For this review, take the finished solid that the model builds, in its own axes (mm). A direction names the side the tool comes from. Round coordinates to 2 decimals unless told otherwise and drop trailing zeros. Write each loop counter-clockwise with the first axis right and the second up, starting at its lowest first coordinate (ties: lowest second). Pieces come first, ordered by that corner, then holes.
from build123d import *

# Parameters (mm, degrees)
BOSS_EXTRUDE1_DEPTH = 60
BOSS_EXTRUDE2_DEPTH = 42
CUT_EXTRUDE1_DEPTH  = 42
SKETCH4_R           = 15
SKETCH4_R_2         = 10
BOSS_EXTRUDE4_DEPTH = 18
CUT_EXTRUDE2_START  = -10
SKETCH4_2_R         = 10
CUT_EXTRUDE2_DEPTH  = 10
CUT_EXTRUDE3_START  = -127
SKETCH5_W           = 40
SKETCH5_H           = 20
CUT_EXTRUDE3_DEPTH  = 127
SKETCH6_R           = 6.5
CUT_EXTRUDE4_DEPTH  = 183
SKETCH7_R           = 4
CUT_EXTRUDE5_DEPTH  = 245
FILLET1_R           = 3
FILLET2_R           = 5
BOSS_EXTRUDE6_DEPTH = 22


with BuildPart() as part:
    # Sketch1 → Boss-Extrude1 (new body)
    with BuildSketch(Plane.XY):
        Polygon((170, 20), (130, 20), (0, 20), (0, 0), (170, 0), align=None)
    extrude(amount=BOSS_EXTRUDE1_DEPTH)

    # Sketch1<3> → Boss-Extrude2 (add)
    with BuildSketch(Plane.XY):
        with BuildLine():
            Line((35, 60), (35, 20))
            Line((35, 20), (45, 20))
            Line((45, 20), (45, 60))
            ThreePointArc((45, 60), (49.292505485, 81.301408404), (61.5, 99.277856357))
            ThreePointArc((61.5, 99.277856357), (66.936491673, 100.316914371), (70, 95.707142143))
            Line((70, 95.707142143), (70, 20))
            Line((70, 20), (100, 20))
            Line((100, 20), (78, 45))
            Line((78, 45), (78, 85))
            Line((78, 85), (130, 85))
            Line((130, 85), (130, 157))
            Line((130, 157), (115, 157))
            Line((115, 157), (115, 175))
            Line((115, 175), (85, 175))
            Line((85, 175), (85, 157))
            Line((85, 157), (70, 157))
            Line((70, 157), (70, 117.662812973))
            ThreePointArc((70, 117.662812973), (44.434723073, 93.726843908), (35, 60))
        make_face()
        Polygon((100, 20), (130, 20), (130, 45), (122, 45), align=None)
    extrude(amount=BOSS_EXTRUDE2_DEPTH)

    # Sketch3 → Cut-Extrude1 (cut)
    with BuildSketch(Plane(origin=(115, 0, 0), x_dir=(0, 0, -1), z_dir=(1, 0, 0))):
        Polygon((-42, 157), (7.234036257, 157), (7.234036257, 179.627454065), (-54.634398112, 179.627454065), (-54.634398112, 157), align=None)
    extrude(amount=-CUT_EXTRUDE1_DEPTH, mode=Mode.SUBTRACT)

    # Sketch4 → Boss-Extrude4 (add)
    with BuildSketch(Plane(origin=(0, 157, 0), x_dir=(1, 0, 0), z_dir=(0, 1, 0))):
        with Locations((100, -21)):
            Circle(SKETCH4_R)
        with Locations(Location((100, -21, 0), (0, 0, 180))):
            Circle(SKETCH4_R_2, mode=Mode.SUBTRACT)
    extrude(amount=BOSS_EXTRUDE4_DEPTH)

    # Sketch4<2> → Cut-Extrude2 (cut)
    with BuildSketch(Plane(origin=(0, 157, 0), x_dir=(1, 0, 0), z_dir=(0, 1, 0)).offset(CUT_EXTRUDE2_START)):
        with Locations(Location((100, -21, 0), (0, 0, 180))):
            Circle(SKETCH4_2_R)
    extrude(amount=CUT_EXTRUDE2_DEPTH, mode=Mode.SUBTRACT)

    # Sketch5 → Cut-Extrude3 (cut)
    with BuildSketch(Plane(origin=(0, 147, 0), x_dir=(1, 0, 0), z_dir=(0, 1, 0)).offset(CUT_EXTRUDE3_START)):
        with Locations((100, -21)):
            Rectangle(SKETCH5_W, SKETCH5_H)
    extrude(amount=CUT_EXTRUDE3_DEPTH, mode=Mode.SUBTRACT)

    # Sketch6 → Cut-Extrude4 (cut)
    with BuildSketch(Plane(origin=(0, 20, 0), x_dir=(1, 0, 0), z_dir=(0, 1, 0))):
        with Locations(Location((15, -30, 0), (0, 0, 180))):
            Circle(SKETCH6_R)
        with Locations(Location((155, -30, 0), (0, 0, 180))):
            Circle(SKETCH6_R)
    extrude(amount=-CUT_EXTRUDE4_DEPTH, mode=Mode.SUBTRACT)

    # Sketch7 → Cut-Extrude5 (cut)
    with BuildSketch(Plane(origin=(130, 0, 0), x_dir=(0, 0, -1), z_dir=(1, 0, 0))):
        with Locations((-20, 140)):
            Circle(SKETCH7_R)
    extrude(amount=-CUT_EXTRUDE5_DEPTH, mode=Mode.SUBTRACT)

    # Fillet1
    # the kernel refuses this fillet: 3 mm, written as the material it adds along each edge
    with BuildSketch(Plane(origin=(100, 20, 42), x_dir=(0, 0, 1), z_dir=(1, 0, 0))) as fillet1_piece_1_section:
        with BuildLine():
            CenterArc((FILLET1_R, -FILLET1_R), FILLET1_R, 90, 90)
            Line((0, -FILLET1_R), (0, 0))
            Line((0, 0), (FILLET1_R, 0))
        make_face()
    fillet1_piece_1 = extrude(amount=30, mode=Mode.PRIVATE)
    fillet1_piece_1 = split(fillet1_piece_1, bisect_by=Plane(origin=(107.006094621, 27.96147116, 42.686468699), z_dir=(0.7507135169227557, -0.6606278948920244, 0)), keep=Keep.TOP, mode=Mode.PRIVATE)
    add(fillet1_piece_1)
    with BuildSketch(Plane(origin=(78, 85, 0), x_dir=(0, -1, 0), z_dir=(0, 0, 1))) as fillet1_piece_2_section:
        with BuildLine():
            CenterArc((FILLET1_R, FILLET1_R), FILLET1_R, 180, 90)
            Line((0, FILLET1_R), (0, 0))
            Line((0, 0), (FILLET1_R, 0))
        make_face()
    fillet1_piece_2 = extrude(amount=42, mode=Mode.PRIVATE)
    fillet1_piece_2 = split(fillet1_piece_2, bisect_by=Plane(origin=(78.588320005, 84.284989696, 11), z_dir=(0, 0, -1)), keep=Keep.TOP, mode=Mode.PRIVATE)
    fillet1_piece_2 = split(fillet1_piece_2, bisect_by=Plane(origin=(80, 84.284989696, 5.5), z_dir=(-1, 0, 0)), keep=Keep.TOP, mode=Mode.PRIVATE)
    add(fillet1_piece_2)
    with BuildSketch(Plane(origin=(78, 85, 0), x_dir=(0, -1, 0), z_dir=(0, 0, 1))) as fillet1_piece_3_section:
        with BuildLine():
            CenterArc((FILLET1_R, FILLET1_R), FILLET1_R, 180, 90)
            Line((0, FILLET1_R), (0, 0))
            Line((0, 0), (FILLET1_R, 0))
        make_face()
    fillet1_piece_3 = extrude(amount=42, mode=Mode.PRIVATE)
    fillet1_piece_3 = split(fillet1_piece_3, bisect_by=Plane(origin=(80.37802851, 84.990607918, 11), z_dir=(0, 0, -1)), keep=Keep.TOP, mode=Mode.PRIVATE)
    fillet1_piece_3 = split(fillet1_piece_3, bisect_by=Plane(origin=(80, 84.990607918, 5.5), z_dir=(1, 0, 0)), keep=Keep.TOP, mode=Mode.PRIVATE)
    add(fillet1_piece_3)
    with BuildSketch(Plane(origin=(78, 85, 0), x_dir=(0, -1, 0), z_dir=(0, 0, 1))) as fillet1_piece_4_section:
        with BuildLine():
            CenterArc((FILLET1_R, FILLET1_R), FILLET1_R, 180, 90)
            Line((0, FILLET1_R), (0, 0))
            Line((0, 0), (FILLET1_R, 0))
        make_face()
    fillet1_piece_4 = extrude(amount=42, mode=Mode.PRIVATE)
    fillet1_piece_4 = split(fillet1_piece_4, bisect_by=Plane(origin=(78.588320005, 84.284989696, 11), z_dir=(0, 0, 1)), keep=Keep.TOP, mode=Mode.PRIVATE)
    fillet1_piece_4 = split(fillet1_piece_4, bisect_by=Plane(origin=(80, 84.284989696, 21), z_dir=(-1, 0, 0)), keep=Keep.TOP, mode=Mode.PRIVATE)
    fillet1_piece_4 = split(fillet1_piece_4, bisect_by=Plane(origin=(78.588320005, 84.284989696, 31), z_dir=(0, 0, -1)), keep=Keep.TOP, mode=Mode.PRIVATE)
    add(fillet1_piece_4)
    with BuildSketch(Plane(origin=(78, 85, 0), x_dir=(0, -1, 0), z_dir=(0, 0, 1))) as fillet1_piece_5_section:
        with BuildLine():
            CenterArc((FILLET1_R, FILLET1_R), FILLET1_R, 180, 90)
            Line((0, FILLET1_R), (0, 0))
            Line((0, 0), (FILLET1_R, 0))
        make_face()
    fillet1_piece_5 = extrude(amount=42, mode=Mode.PRIVATE)
    fillet1_piece_5 = split(fillet1_piece_5, bisect_by=Plane(origin=(80, 84.284989696, 36.5), z_dir=(-1, 0, 0)), keep=Keep.TOP, mode=Mode.PRIVATE)
    fillet1_piece_5 = split(fillet1_piece_5, bisect_by=Plane(origin=(78.588320005, 84.284989696, 31), z_dir=(0, 0, 1)), keep=Keep.TOP, mode=Mode.PRIVATE)
    add(fillet1_piece_5)
    with BuildSketch(Plane(origin=(78, 85, 0), x_dir=(0, -1, 0), z_dir=(0, 0, 1))) as fillet1_piece_6_section:
        with BuildLine():
            CenterArc((FILLET1_R, FILLET1_R), FILLET1_R, 180, 90)
            Line((0, FILLET1_R), (0, 0))
            Line((0, 0), (FILLET1_R, 0))
        make_face()
    fillet1_piece_6 = extrude(amount=42, mode=Mode.PRIVATE)
    fillet1_piece_6 = split(fillet1_piece_6, bisect_by=Plane(origin=(80, 84.990607918, 36.5), z_dir=(1, 0, 0)), keep=Keep.TOP, mode=Mode.PRIVATE)
    fillet1_piece_6 = split(fillet1_piece_6, bisect_by=Plane(origin=(80.37802851, 84.990607918, 31), z_dir=(0, 0, 1)), keep=Keep.TOP, mode=Mode.PRIVATE)
    add(fillet1_piece_6)
    with BuildSketch(Plane(origin=(130, 20, 0), x_dir=(1, 0, 0), z_dir=(0, 0, 1))) as fillet1_piece_7:
        with BuildLine():
            CenterArc((FILLET1_R, FILLET1_R), FILLET1_R, 180, 90)
            Line((0, FILLET1_R), (0, 0))
            Line((0, 0), (FILLET1_R, 0))
        make_face()
    extrude(amount=42)
    with BuildSketch(Plane(origin=(70, 20, 42), x_dir=(0, 0, 1), z_dir=(1, 0, 0))) as fillet1_piece_8_section:
        with BuildLine():
            CenterArc((FILLET1_R, -FILLET1_R), FILLET1_R, 90, 90)
            Line((0, -FILLET1_R), (0, 0))
            Line((0, 0), (FILLET1_R, 0))
        make_face()
    fillet1_piece_8 = extrude(amount=30, mode=Mode.PRIVATE)
    fillet1_piece_8 = split(fillet1_piece_8, bisect_by=Plane(origin=(92.993905379, 27.96147116, 42.686468699), z_dir=(-0.7507135169227557, -0.6606278948920244, 0)), keep=Keep.TOP, mode=Mode.PRIVATE)
    add(fillet1_piece_8)
    with BuildSketch(Plane(origin=(35, 20, 0), x_dir=(-1, 0, 0), z_dir=(0, 0, 1))) as fillet1_piece_9:
        with BuildLine():
            CenterArc((FILLET1_R, -FILLET1_R), FILLET1_R, 90, 90)
            Line((0, -FILLET1_R), (0, 0))
            Line((0, 0), (FILLET1_R, 0))
        make_face()
    extrude(amount=42)
    with BuildSketch(Plane(origin=(35, 20, 42), x_dir=(0, 0, 1), z_dir=(1, 0, 0))) as fillet1_piece_10:
        with BuildLine():
            CenterArc((FILLET1_R, -FILLET1_R), FILLET1_R, 90, 90)
            Line((0, -FILLET1_R), (0, 0))
            Line((0, 0), (FILLET1_R, 0))
        make_face()
    extrude(amount=10)
    with BuildSketch(Plane(origin=(130, 20, 0), x_dir=(1, 0, 0), z_dir=(0, 0, 1))) as fillet1_piece_11a_section:
        with BuildLine():
            CenterArc((FILLET1_R, FILLET1_R), FILLET1_R, 180, 90)
            Line((0, FILLET1_R), (0, 0))
            Line((0, 0), (FILLET1_R, 0))
        make_face()
    fillet1_piece_11a = extrude(amount=49.5, mode=Mode.PRIVATE)
    fillet1_piece_11a = split(fillet1_piece_11a, bisect_by=Plane(origin=(130.679185343, 20.679185343, 42), z_dir=(0, 0, 1)), keep=Keep.TOP, mode=Mode.PRIVATE)
    with BuildSketch(Plane(origin=(100, 20, 42), x_dir=(0, 0, 1), z_dir=(1, 0, 0))) as fillet1_piece_11b_section:
        with BuildLine():
            CenterArc((FILLET1_R, -FILLET1_R), FILLET1_R, 90, 90)
            Line((0, -FILLET1_R), (0, 0))
            Line((0, 0), (FILLET1_R, 0))
        make_face()
    fillet1_piece_11b = extrude(amount=37.5, mode=Mode.PRIVATE)
    fillet1_piece_11b = split(fillet1_piece_11b, bisect_by=Plane(origin=(130, 20.679185343, 42.679185343), z_dir=(1, 0, 0)), keep=Keep.TOP, mode=Mode.PRIVATE)
    fillet1_piece_11 = fillet1_piece_11a & fillet1_piece_11b
    add(fillet1_piece_11)
    with BuildSketch(Plane(origin=(35, 20, 0), x_dir=(-1, 0, 0), z_dir=(0, 0, 1))) as fillet1_piece_12a_section:
        with BuildLine():
            CenterArc((FILLET1_R, -FILLET1_R), FILLET1_R, 90, 90)
            Line((0, -FILLET1_R), (0, 0))
            Line((0, 0), (FILLET1_R, 0))
        make_face()
    fillet1_piece_12a = extrude(amount=49.5, mode=Mode.PRIVATE)
    fillet1_piece_12a = split(fillet1_piece_12a, bisect_by=Plane(origin=(34.320814657, 20.679185343, 42), z_dir=(0, 0, 1)), keep=Keep.TOP, mode=Mode.PRIVATE)
    with BuildSketch(Plane(origin=(27.5, 20, 42), x_dir=(0, 0, 1), z_dir=(1, 0, 0))) as fillet1_piece_12b_section:
        with BuildLine():
            CenterArc((FILLET1_R, -FILLET1_R), FILLET1_R, 90, 90)
            Line((0, -FILLET1_R), (0, 0))
            Line((0, 0), (FILLET1_R, 0))
        make_face()
    fillet1_piece_12b = extrude(amount=17.5, mode=Mode.PRIVATE)
    fillet1_piece_12b = split(fillet1_piece_12b, bisect_by=Plane(origin=(35, 20.679185343, 42.679185343), z_dir=(-1, 0, 0)), keep=Keep.TOP, mode=Mode.PRIVATE)
    fillet1_piece_12 = fillet1_piece_12a & fillet1_piece_12b
    add(fillet1_piece_12)
    # the kernel refuses this fillet: 3 mm, written as the material it takes off along each edge
    with BuildSketch(Plane(origin=(70, 157, -7.5), x_dir=(1, 0, 0), z_dir=(0, 0, 1))) as fillet1_2_piece_1:
        with BuildLine():
            CenterArc((FILLET1_R, -FILLET1_R), FILLET1_R, 90, 90)
            Line((0, -FILLET1_R), (0, 0))
            Line((0, 0), (FILLET1_R, 0))
        make_face()
    extrude(amount=57, mode=Mode.SUBTRACT)
    with BuildSketch(Plane(origin=(130, 157, -7.5), x_dir=(-1, 0, 0), z_dir=(0, 0, 1)), Plane(origin=(130, 85, -7.5), x_dir=(0, 1, 0), z_dir=(0, 0, 1))) as fillet1_2_piece_2:
        with BuildLine():
            CenterArc((FILLET1_R, FILLET1_R), FILLET1_R, 180, 90)
            Line((0, FILLET1_R), (0, 0))
            Line((0, 0), (FILLET1_R, 0))
        make_face()
    extrude(amount=57, mode=Mode.SUBTRACT)

    # Fillet2
    fillet2_edges = [part.edges().sort_by_distance(p)[0] for p in [
        (0, 10, 60),
        (170, 10, 60),
        (170, 10, 0),
        (0, 10, 0),
    ]]
    fillet(fillet2_edges, radius=FILLET2_R)

    # Sketch8 → Boss-Extrude6 (add)
    with BuildSketch(Plane(origin=(0, 0, 10), x_dir=(-1, 0, 0), z_dir=(0, 0, -1))):
        with BuildLine():
            ThreePointArc((-45, 60), (-49.292505485, 81.301408404), (-61.5, 99.277856357))
            ThreePointArc((-61.5, 99.277856357), (-66.936491673, 100.316914371), (-70, 95.707142143))
            Line((-70, 95.707142143), (-70, 20))
            Line((-70, 20), (-45, 20))
            Line((-45, 20), (-45, 60))
        make_face()
    extrude(amount=-BOSS_EXTRUDE6_DEPTH)


solid = part.part
(1) For faces 1 (the face through (88, 29, 11)), 2 (the face through (110, 161, 21)), 3 (the face through (70, 57, 5)), list the 3-axis set-ups (+Z, -Z, +X, -X, +Y, -Y) from which the entire face can be reached by the end or side of a thin tool; tool diameter is ignored.
Geometry check:
face 1: none
face 2: +Y
face 3: -Z
(2) We need section B-B, the plane y = 110. Give the boundary of the cut face in (x, z).
Geometry check:
outline: (58.47, 0) - (130, 0) - (130, 42) - (58.47, 42) - close; hole (80, 11) - (120, 11) - (120, 31) - (80, 31) - close
(3) We need section A-A, the plane y = 37. Give the boundary of the cut face in (x, z), and give its area (3 significant figures).
Geometry check:
outline: (35, 0) - (45, 0) - (45, 10) - (70, 10) - (70, 0) - (85.04, 0) - (85.04, 11) - (80, 11) - (80, 31) - (85.04, 31) - (85.04, 42) - (70, 42) - (70, 32) - (45, 32) - (45, 42) - (35, 42) - close; (114.96, 0) - (130, 0) - (130, 42) - (114.96, 42) - (114.96, 31) - (120, 31) - (120, 11) - (114.96, 11) - close
area: 2,030 mm2
(4) We need section C-C, the plane y = 140. Give the boundary of the cut face in (x, z), and give its area (3 significant figures).
Geometry check:
outline: (70, 0) - (130, 0) - (130, 16) - (120, 16) - (120, 11) - (80, 11) - (80, 16) - (70, 16) - close; (70, 24) - (80, 24) - (80, 31) - (120, 31) - (120, 24) - (130, 24) - (130, 42) - (70, 42) - close
area: 1,560 mm2
(5) We need section D-D, the plane x = 145. Give the boundary of the cut face in (y, z), and give its area (3 significant figures).
Geometry check:
outline: (0, 0) - (20, 0) - (20, 60) - (0, 60) - close
area: 1,200 mm2
(6) Mouldability with a two-part tool opening along Y and no side actions: class faces 4 (the face through (130, 121, 21)), 5 (the face through (120, 116, 21)), 6 (the face through (84, 0, 30)) as pulls with the +Y half, pulls with the -Y half, needs draft (parallel to the pull), parting line crosses it, or undercut.
Geometry check:
face 4: needs draft
face 5: undercut
face 6: pulls with the -Y half
(7) For pin 1 Ø21 at (y, z) = (133, 25) entering from +X; pin 2 Ø1 at (y, z) = (53.5, 36.5) entering from -X; pin 3 Ø1 at (x, y) = (118, 41.5) entering from -Z; pin 4 Ø22 at (x, y) = (90.5, 34) entering from +Z, all flat-tipped, find the tip position at first contact; note any pin that passes through.
Geometry check:
pin 1: stops at x = 130
pin 2: stops at x = 35
pin 3: passes through
pin 4: stops at z = 42
(8) For line 1 along Y through (x, z) = (123.5, 20); line 2 along Z through (x, y) = (15, 12.25); line 3 along X through (y, z) = (138.5, 26), list the stretches that pass through material, from the lowest coordinate up.
Geometry check:
line 1: y = 0 to 45, 85 to 136, 144 to 157
line 2: z = 0 to 23.5, 36.5 to 60
line 3: x = 70 to 80, 120 to 130
